Part model, mm, in its own coordinate system. Give positions to 0.01 mm unless a question says otherwise; leave off trailing zeros. Write each loop counter-clockwise with the first axis right and the second up, starting at its lowest first coordinate (ties: lowest second). Pieces come first, ordered by that corner, then holes. Notation, with made-up numbers: M -1,58.25 L 34,58.25 A19 cw 34,62.25 Z; hole C -28,-7.75 d4. An arc over 180 degrees is marked long. Answer as CSV lines item,"result". Start each with the question number.
Item 1: Two-plate mould, pull along X, no slides. Class faces 1 (the cylindrical face through (10.752, -128.136, 5.07)), 2 (the flat face through (-40, 3, 5)), 3 (the flat face through (40, -3, 5)): +X half, -X half, draft (parallel to the pull), parting line (faces both ways), or undercut.
Item 2: Band-saw the part on B-B, the plane y = -145. List the corners of the cut face in (x, z).
Item 3: Band-saw the part on D-D, the plane z = 4.5. Count the separate pieces of the cut face and the enclosed holes in it, then the cut area to 3 significant figures.
Item 4: Band-saw the part on C-C, the plane x = 7. List the corners of the cut face in (y, z) (3 decimals).
Item 5: Band-saw the part on A-A, the plane x = 27. List the corners of the cut face in (y, z), then the cut area to 3 significant figures.
Item 6: Pin check, flat tips, straight feed: pin 1 (1.9 mm diameter, centred on x = 16, y = -129, fed in from +Z); pin 2 (2.5 mm diameter, centred on x = 16, y = 96, fed in from +Z). Stop position of each tip, or through.
Item 7: Wall check: L1, parallel to X at y = -161, z = 5; L2, parallel to X at y = 47, z = 7.25; L3, parallel to X at y = 83.5, z = 8. Give the ranges that are in metal, low to high. Write a range as from..to.
Autodesk Inventor part; units mm, degrees
ref_plane "YZ Plane" through (0, 0, 0) normal (1, 0, 0) x (0, 1, 0)
ref_plane "XZ Plane" through (0, 0, 0) normal (0, 1, 0) x (-1, 0, 0)
ref_plane "XY Plane" through (0, 0, 0) normal (0, 0, 1) x (1, 0, 0)
sketch "Skizze1" plane through (0, 0, 0) normal (0, 0, 1) x (1, 0, 0)
  line L0 (40, 180) -> (-40, 180)
  line L1 (-40, 180) -> (-40, -180)
  line L2 (-40, -180) -> (40, -180)
  line L3 (40, -180) -> (40, 180)
  line L4 (40, 180) -> (-40, -180) construction
  line L5 (-40, 180) -> (40, -180) construction
  point P0 (0, 0)
  dimension "d0" = 80
  dimension "d1" = 360
extrude "Extrusion1" add sketch "Skizze1" along normal blind 10
hole "Bohrung3" at (27, -110, 10) direction (0, 0, -1) diameter 6 end through all
sketch "Skizze2" plane through (0, 0, 10) normal (0, 0, 1) x (1, 0, 0)
  line L0 (40, 180) -> (-40, 180)
  circle A0 centre (0, 130) radius 20
  point P0 (0, 0)
  dimension "d40" = 40
  dimension "d41" = 50
extrude "Extrusion2" cut sketch "Skizze2" against normal blind 10
sketch "Skizze3" plane through (0, 0, 10) normal (0, 0, 1) x (1, 0, 0)
  circle A0 centre (0, 130) radius 20
  line L0 (16, 114) -> (-16, 114)
  line L1 (-16, 114) -> (-16, 146)
  line L2 (-16, 146) -> (16, 146)
  line L3 (16, 146) -> (16, 114)
  line L4 (16, 114) -> (-16, 146) construction
  line L5 (-16, 114) -> (16, 146) construction
  dimension "d45" = 32
hole "Bohrung4" at (16, 114, 10) at (-16, 114, 10) at (-16, 146, 10) at (16, 146, 10) direction (0, 0, -1) diameter 3.242 depth 8 tip angle 118
pattern_linear "Rechteckige Anordnung3" count 5 spacing 50 along (0, -1, 0) of "Extrusion2", "Bohrung4"
pattern_linear "Rechteckige Anordnung4" count 2 spacing 275 along (0, -1, 0) of "Extrusion2", "Bohrung4"
properties part number "Tunel_LidWithFanHoles" material "Polycarbonat, klar"
Output:
1,face 1,"undercut"
1,face 2,"-X half"
1,face 3,"+X half"
2,outline,"M -40,0 L -20,0 L -20,10 L -40,10 Z; M 20,0 L 40,0 L 40,10 L 20,10 Z"
3,separate pieces,"1"
3,enclosed holes,"31"
3,area,"21,000 mm²"
4,outline,"M -180,0 L -163.735,0 L -163.735,10 L -180,10 Z; M -126.265,0 L -88.735,0 L -88.735,10 L -126.265,10 Z; M -51.265,0 L -38.735,0 L -38.735,10 L -51.265,10 Z; M -1.265,0 L 11.265,0 L 11.265,10 L -1.265,10 Z; M 48.735,0 L 61.265,0 L 61.265,10 L 48.735,10 Z; M 98.735,0 L 111.265,0 L 111.265,10 L 98.735,10 Z; M 148.735,0 L 180,0 L 180,10 L 148.735,10 Z"
5,outline,"M -180,0 L -113,0 L -113,10 L -180,10 Z; M -107,0 L 180,0 L 180,10 L -107,10 Z"
5,area,"3,540 mm²"
6,pin 1,"z = 1.6"
6,pin 2,"z = 1.78"
7,L1,"-40..-17.62, -14.38..-12, 12..14.38, 17.62..40"
7,L2,"-40..-17.28, -14.72..-10.54, 10.54..14.72, 17.28..40"
7,L3,"-40..-19.69, 19.69..40"
